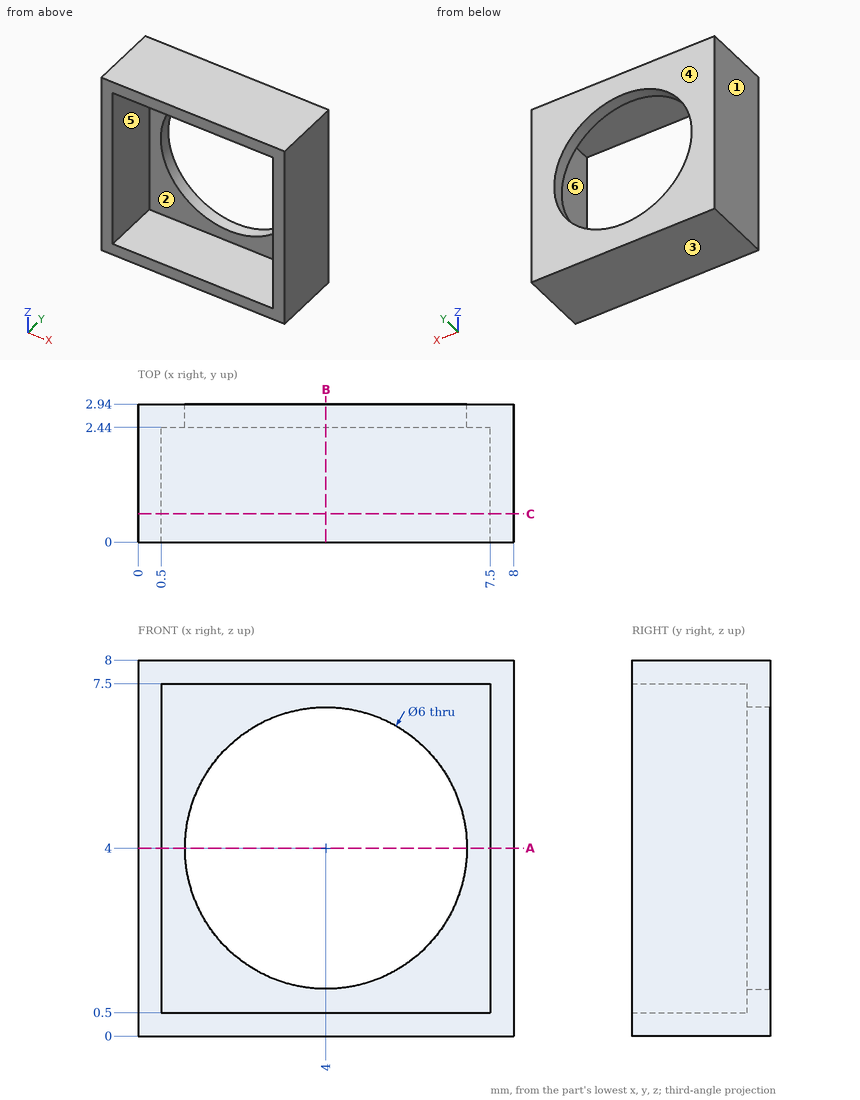
Job drawing, mm, ordinate dimensions from the low corner. One solid piece. A direction names the side the tool comes from. Coordinates: 2 decimals unless noted, no trailing zeros. Order: outer loops, then holes, each group sorted by start corner. A loop starts at its lowest first (then second) coordinate and runs counter-clockwise, first axis right, second up. Notation, with made-up numbers: (-40, 54.25) -> (-14, 54.25) arc R9 ccw to (-14, 67.25) -> close; hole circle Ø2 at (55, -17.5). An arc over 180 degrees is marked (long way). Answer in a Markdown table with one row per item. Add a question column.
Q1. Band-saw the part on B-B, the plane x = 4. List the corners of the cut face in (y, z), then the cut area to 3 significant figures.
Q2. Wall check: line 1 along X through (y, z) = (1.3, 2); line 2 along X through (y, z) = (2.6, 4). Give the ranges that are in metal, low to high. Write a range as [from, to].
Q3. Mould opens along Z. For the marked faces 3, 4, 5 and 6 say: +Z half, -Z half, draft (parallel to the pull), parting line (faces both ways), or undercut.
Q4. Which spindle directions (+Z, -Z, +X, -X, +Y, -Y) get a long thin tool onto all of the face, cutting with end or side? Do the marked faces 1 and 2. Say none if no direction does.
Q5. Band-saw the part on A-A, the plane z = 4. List the corners of the cut face in (x, y).
Q6. Band-saw the part on C-C, the plane y = 0.6. List the corners of the cut face in (x, z).
Answers follow:
| question | item | result |
|---|---|---|
| 1 | outline | (0, 0) -> (2.94, 0) -> (2.94, 1) -> (2.44, 1) -> (2.44, 0.5) -> (0, 0.5) -> close; (0, 7.5) -> (2.44, 7.5) -> (2.44, 7) -> (2.94, 7) -> (2.94, 8) -> (0, 8) -> close |
| 1 | area | 3.44 mm^2 |
| 2 | line 1 | [0, 0.5], [7.5, 8] |
| 2 | line 2 | [0, 1], [7, 8] |
| 3 | face 3 | -Z half |
| 3 | face 4 | draft |
| 3 | face 5 | undercut |
| 3 | face 6 | undercut |
| 4 | face 1 | +Z, -Z, -X, +Y, -Y |
| 4 | face 2 | -Y |
| 5 | outline | (0, 0) -> (0.5, 0) -> (0.5, 2.44) -> (1, 2.44) -> (1, 2.94) -> (0, 2.94) -> close; (7, 2.44) -> (7.5, 2.44) -> (7.5, 0) -> (8, 0) -> (8, 2.94) -> (7, 2.94) -> close |
| 6 | outline | (0, 0) -> (8, 0) -> (8, 8) -> (0, 8) -> close; hole (0.5, 0.5) -> (7.5, 0.5) -> (7.5, 7.5) -> (0.5, 7.5) -> close |
